from build123d import *

# Parameters (mm, degrees)
SKETCH1_W           = 28.956
SKETCH1_H           = 15.24
SKETCH1_R           = 1.6002
BOSS_EXTRUDE1_DEPTH = 6.35
SKETCH2_W           = 28.956
SKETCH2_H           = 19.05
SKETCH2_R           = 2.413
BOSS_EXTRUDE2_DEPTH = 5.08
FILLET1_R           = 2.54


with BuildPart() as part:
    # Sketch1 → Boss-Extrude1 (new body)
    with BuildSketch(Plane(origin=(0, 0, 0), x_dir=(1, 0, 0), z_dir=(0, 1, 0))):
        Rectangle(SKETCH1_W, SKETCH1_H)
        with Locations(Location((-11.176, 5.207, 0), (0, 0, 270))):
            Circle(SKETCH1_R, mode=Mode.SUBTRACT)
        with Locations(Location((11.176, -5.207, 0), (0, 0, 270))):
            Circle(SKETCH1_R, mode=Mode.SUBTRACT)
    extrude(amount=-BOSS_EXTRUDE1_DEPTH)

    # Sketch2 → Boss-Extrude2 (add)
    with BuildSketch(Plane(origin=(0, 0, -7.62), x_dir=(-1, 0, 0), z_dir=(0, 0, -1))):
        with Locations((0, -15.875)):
            Rectangle(SKETCH2_W, SKETCH2_H)
        with Locations((-6.35, -15.875)):
            Circle(SKETCH2_R, mode=Mode.SUBTRACT)
        with Locations((6.35, -15.875)):
            Circle(SKETCH2_R, mode=Mode.SUBTRACT)
    extrude(amount=-BOSS_EXTRUDE2_DEPTH)

    # Fillet1
    fillet1_edges = [part.edges().sort_by_distance(p)[0] for p in [
        (0, -6.35, -2.54),
        (14.478, -25.4, -5.08),
        (-14.478, -25.4, -5.08),
        (14.478, -3.175, 7.62),
        (-14.478, -3.175, 7.62),
    ]]
    fillet(fillet1_edges, radius=FILLET1_R)


solid = part.part
Check sheet for the modelled part. Datum: model origin and axes. Units: mm. A direction names the side the tool comes from. Round coordinates to 2 decimals unless told otherwise and drop trailing zeros. Loops run counter-clockwise (first coordinate to the right, second up) from the corner with the lowest first, then second, coordinate; pieces in that order, holes last.
1. Sectioned sample at A-A on x = -6.35. Record the boundary of the cut face in (y, z), and give its area (3 significant figures).
2. Gauge pin test, flat ends, axial feed: pin 1 Ø12 at (x, y) = (1, -16.5) entering from +Z; pin 2 Ø6 at (x, z) = (3.5, 2.5) entering from -Y; pin 3 Ø1.9 at (x, z) = (-11.176, -5.207) entering from +Y. Record the tip position at first contact, or that the pin passes through.
3. Scan lines: probe 1 along X at (y, z) = (-14, -3.25); probe 2 along Y at (x, z) = (6.35, -4.5); probe 3 along Y at (x, z) = (3.75, 3.5). Record each from-to range of solid material in increasing order.
4. Sectioned sample at C-C on z = -5.75. Record the boundary of the cut face in (x, y) (3 decimals), and give its area (3 significant figures).
5. Mould release check, pull along Y, two halves, no side actions. Record for faces 1 (the cylindrical face through (-13.75, -24.64, -5.04)), 2 (the cylindrical face through (8.265, -17.343, -5.116)), 3 (the cylindrical face through (9.76, -3.13, 5.95)): released by +Y, released by -Y, zero draft, split by the parting line, or undercut.
6. Set-up check for faces 4 (the flat face through (0, -17, -2.54)), 5 (the flat face through (-11, -6.35, -5)), 6 (the flat face through (0, -3, 7.62)): record each of +Z, -Z, +X, -X, +Y, -Y from which the full face is reachable in a straight line by a thin tool's end or side.
7. Sectioned sample at D-D on y = -9.5. Record the boundary of the cut face in (x, z).
8. Sectioned sample at B-B on z = 4.5. Record the boundary of the cut face in (x, y).
Recorded:
1. outline: (-25.4, -7.62) - (-18.29, -7.62) - (-18.29, -2.54) - (-25.4, -2.54) - close; (-13.46, -7.62) - (0, -7.62) - (0, 7.62) - (-6.35, 7.62) - (-6.35, 0) arc R2.54 cw to (-8.89, -2.54) - (-13.46, -2.54) - close
1. area: 170 mm2
2. pin 1: stops at z = -2.54
2. pin 2: stops at y = -6.4
2. pin 3: stops at y = -6.35
3. probe 1: x = -14.48 to -7.87, -4.83 to 4.83, 7.87 to 14.48
3. probe 2: y = -25.4 to -18.29, -13.46 to 0
3. probe 3: y = -6.35 to 0
4. outline: (-14.478, -22.86) arc R2.54 ccw to (-11.938, -25.4) - (11.938, -25.4) arc R2.54 ccw to (14.478, -22.86) - (14.478, 0) - (-9.671, 0) - (-9.671, -6.35) - (-12.681, -6.35) - (-12.681, 0) - (-14.478, 0) - close; hole circle Ø4.826 at (-6.35, -15.875); hole circle Ø4.826 at (6.35, -15.875)
4. area: 677 mm2
5. face 1: released by -Y
5. face 2: undercut
5. face 3: zero draft
6. face 4: +Z, +X, -X, -Y
6. face 5: +Y
6. face 6: +Z, +X, -X, +Y, -Y
7. outline: (-14.48, -7.62) - (14.48, -7.62) - (14.48, -2.54) - (-14.48, -2.54) - close
8. outline: (-14.48, -6.35) - (9.74, -6.35) - (9.74, 0) - (-14.48, 0) - close; (12.61, -6.35) - (14.48, -6.35) - (14.48, 0) - (12.61, 0) - close
